Geometry: final body of the model. Coordinates: model frame, mm. A direction names the side the tool comes from. Give positions to 0.01 mm unless a question says otherwise; leave off trailing zeros. Loops run counter-clockwise (first coordinate to the right, second up) from the corner with the lowest first, then second, coordinate; pieces in that order, holes last.
1. First-contact query: P1, Ø1, axis at x = 8, y = 14.5, coming from the +Z side; P2, Ø1.5, axis at x = 9.5, z = 8, coming from the +Y side; P3, Ø7.5, axis at x = 3.5, z = 7, coming from the -Y side. Flat tips, straight axial feed; report the tip coordinate or a pass-through.
2. Section B-B, the plane z = 11.75. Output: boundary loops of the cut face in (x, y).
3. Section C-C, the plane z = 8.5. Output: boundary loops of the cut face in (x, y).
4. Section D-D, the plane y = 17.25. Output: boundary loops of the cut face in (x, z).
5. Draft query along X for faces 1 (the face through (-12.54, 16.85, 10.27)), 2 (the face through (15, 13, 8)), 3 (the face through (0, 10, 7)). Return one class per face: +X half, -X half, draft (parallel to the pull), parting line (faces both ways), or undercut.
6. Section A-A, the plane y = 13.75. Output: boundary loops of the cut face in (x, z).
7. Access query for faces 4 (the face through (4, 9, 15)), 5 (the face through (-10, 14, 8)), 6 (the face through (10, 3, 7)). Directions: +Z, -Z, +X, -X, +Y, -Y. A direction counts if a zero-diameter tool reaches every point of the face in a straight line with its end or side. Return the directions, or none.
8. Material intervals for line 1 along Y through (x, z) = (-13.2, 7.5); line 2 along X through (y, z) = (17.5, 12); line 3 along Y through (x, z) = (2, 2.5), sorted ascending.
from build123d import *

# Parameters (mm, degrees)
EXTRUDE_1_DEPTH     = 15
EXTRUDE_2_DEPTH     = 5
SKETCH_4_R          = 3
CUT_EXTRUDE_1_DEPTH = 5


with BuildPart() as part:
    # 草图1 → 凸台-拉伸1 (new body)
    with BuildSketch(Plane.XY):
        Polygon((10, 6), (-10, 6), (-10, 0), (-15, 0), (-15, 10), (15, 10), (15, 0), (10, 0), align=None)
    extrude(amount=EXTRUDE_1_DEPTH)

    # 草图2 → 凸台-拉伸2 (add)
    with BuildSketch(Plane.ZY.offset(15)):
        with BuildLine():
            Line((0, 10), (0, 18))
            ThreePointArc((0, 18), (7.5, 25.5), (15, 18))
            Line((15, 18), (15, 10))
            Line((15, 10), (0, 10))
        make_face()
    extrude_2 = extrude(amount=-EXTRUDE_2_DEPTH)

    # 草图4 → 切除-拉伸1 (cut)
    with BuildSketch(Plane.ZY.offset(15)):
        with Locations((7.5, 18)):
            Circle(SKETCH_4_R)
    cut_extrude_1 = extrude(amount=-CUT_EXTRUDE_1_DEPTH, mode=Mode.SUBTRACT)

    # 镜向2: 凸台-拉伸2, 切除-拉伸1 across plane
    add(extrude_2.mirror(Plane(origin=(0, 0, 0), x_dir=(0, 0, 1), z_dir=(1, 0, 0))))
    add(cut_extrude_1.mirror(Plane(origin=(0, 0, 0), x_dir=(0, 0, 1), z_dir=(1, 0, 0))), mode=Mode.SUBTRACT)


solid = part.part
Answers below:
1. P1: passes through
1. P2: stops at y = 25.5
1. P3: stops at y = 6
2. outline: (-15, 0) - (-10, 0) - (-10, 6) - (10, 6) - (10, 0) - (15, 0) - (15, 24.18) - (10, 24.18) - (10, 10) - (-10, 10) - (-10, 24.18) - (-15, 24.18) - close
3. outline: (-15, 0) - (-10, 0) - (-10, 6) - (10, 6) - (10, 0) - (15, 0) - (15, 15.17) - (10, 15.17) - (10, 10) - (-10, 10) - (-10, 15.17) - (-15, 15.17) - close; (-15, 20.83) - (-10, 20.83) - (-10, 25.43) - (-15, 25.43) - close; (10, 20.83) - (15, 20.83) - (15, 25.43) - (10, 25.43) - close
4. outline: (-15, 0) - (-10, 0) - (-10, 4.6) - (-15, 4.6) - close; (-15, 10.4) - (-10, 10.4) - (-10, 15) - (-15, 15) - close; (10, 0) - (15, 0) - (15, 4.6) - (10, 4.6) - close; (10, 10.4) - (15, 10.4) - (15, 15) - (10, 15) - close
5. face 1: draft
5. face 2: +X half
5. face 3: undercut
6. outline: (-15, 0) - (-10, 0) - (-10, 15) - (-15, 15) - close; (10, 0) - (15, 0) - (15, 15) - (10, 15) - close
7. face 4: +Z, +X, -X, +Y, -Y
7. face 5: +Z, -Z, +Y
7. face 6: +Z, -Z, -Y
8. line 1: y = 0 to 15, 21 to 25.5
8. line 2: x = -15 to -10, 10 to 15
8. line 3: y = 6 to 10
